Check sheet for the drawn part. Datum: minimum x, y, z corner. Units: mm. Coordinates: 2 decimals unless noted, no trailing zeros. Order: outer loops, then holes, each group sorted by start corner. A loop starts at its lowest first (then second) coordinate and runs counter-clockwise, first axis right, second up. Notation, with made-up numbers: (-25, -33.5) -> (-8, -33.5) arc R25 ccw to (-8, -10.5) -> close; hole circle Ø2 at (41, -39). An arc over 180 degrees is marked (long way). Answer as CSV lines item,"result".
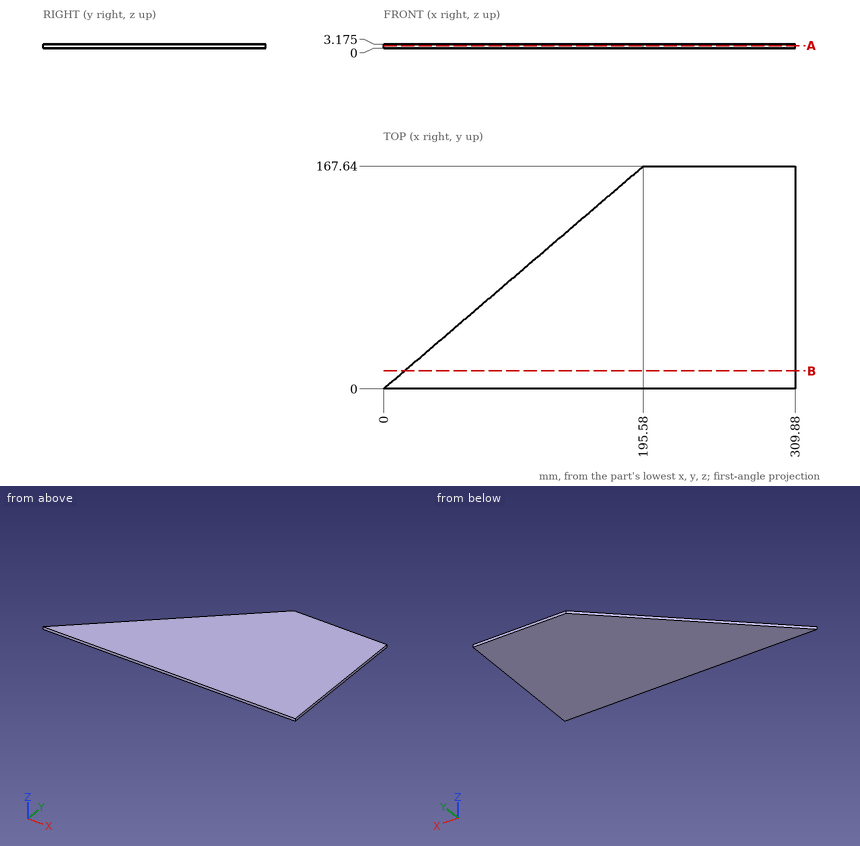
Item 1: Depth check by flat-ended pin: pin 1 Ø1 at (y, z) = (18, 2) entering from -X. Enter the tip coordinate at first touch or a pass-through.
Answer list:
pin 1,"x = 20.42"
Item 2: Thickness scan on line 1 (Y direction, x = 77, z = 2.95); line 2 (X direction, y = 17, z = 1.2); line 3 (X direction, y = 122, z = 2.7). Record the ranges inside material, lowest first.
Answer list:
line 1,"0 to 66"
line 2,"19.83 to 309.88"
line 3,"142.33 to 309.88"
Item 3: Section check B-B, the plane y = 13.5. Record the boundary of the cut face in (x, z) (3 decimals), plus the area to 3 significant figures.
Answer list:
outline,"(15.75, 0) -> (309.88, 0) -> (309.88, 3.175) -> (15.75, 3.175) -> close"
area,"934 mm2"
Item 4: Section check A-A, the plane z = 2. Record the boundary of the cut face in (x, y).
Answer list:
outline,"(0, 0) -> (309.88, 0) -> (309.88, 167.64) -> (195.58, 167.64) -> close"
